Model file for the job. Use its own axes, mm. A direction names the side the tool comes from. Round coordinates to 2 decimals unless told otherwise and drop trailing zeros. Write each loop counter-clockwise with the first axis right and the second up, starting at its lowest first coordinate (ties: lowest second). Pieces come first, ordered by that corner, then holes. Notation, with made-up numbers: (52.5, 71.25) - (57.5, 71.25) arc R13 ccw to (57.5, 94.25) - close; hole circle Ø11 at (12, 2.25). An arc over 180 degrees is marked (long way). One line per item, written item: value.
from build123d import *

# Parameters (mm, degrees)
SKETCH1_R           = 3.4925
BOSS_EXTRUDE1_DEPTH = 25.4
SKETCH2_R           = 1.778
CUT_EXTRUDE1_DEPTH  = 54.415541746
FILLET2_R           = 6.35
FILLET1_R           = 6.35


with BuildPart() as part:
    # Sketch1 → Boss-Extrude1 (new body)
    with BuildSketch(Plane.XY):
        Polygon((0, 0), (44.45, 0), (44.45, 6.35), (31.75, 6.35), (31.75, 21.59), (12.7, 21.59), (12.7, 6.35), (0, 6.35), align=None)
        with Locations((22.225, 13.97)):
            Circle(SKETCH1_R, mode=Mode.SUBTRACT)
    extrude(amount=BOSS_EXTRUDE1_DEPTH)

    # Sketch2 → Cut-Extrude1 (cut, through all)
    with BuildSketch(Plane(origin=(0, 6.35, 0), x_dir=(1, 0, 0), z_dir=(0, 1, 0))):
        with Locations(Location((6.35, -6.35, 0), (0, 0, 270))):
            Circle(SKETCH2_R)
        with Locations(Location((6.35, -19.05, 0), (0, 0, 270))):
            Circle(SKETCH2_R)
        with Locations(Location((38.1, -6.35, 0), (0, 0, 270))):
            Circle(SKETCH2_R)
        with Locations(Location((38.1, -19.05, 0), (0, 0, 270))):
            Circle(SKETCH2_R)
    extrude(amount=-CUT_EXTRUDE1_DEPTH, mode=Mode.SUBTRACT)

    # Fillet2
    fillet2_edges = [part.edges().sort_by_distance(p)[0] for p in [
        (12.7, 21.59, 12.7),
        (31.75, 21.59, 12.7),
    ]]
    fillet(fillet2_edges, radius=FILLET2_R)

    # Fillet1
    fillet1_edges = [part.edges().sort_by_distance(p)[0] for p in [
        (44.45, 3.175, 0),
        (0, 3.175, 0),
        (44.45, 3.175, 25.4),
        (0, 3.175, 25.4),
    ]]
    fillet(fillet1_edges, radius=FILLET1_R)


solid = part.part
1. Wall check: probe 1 along Z at (x, y) = (38, 1); probe 2 along X at (y, z) = (3.75, 6.35); probe 3 along Z at (x, y) = (5, 3.25). Give the ranges that are in metal, low to high. Write a range as [from, to].
Report:
probe 1: [0, 4.57], [8.13, 17.27], [20.83, 25.4]
probe 2: [0, 4.57], [8.13, 36.32], [39.88, 44.45]
probe 3: [0.15, 5.19], [7.51, 17.89], [20.21, 25.25]
2. Band-saw the part on D-D on x = 5.5. Write the cut outline in (y, z).
Report:
outline: (0, 0.06) - (6.35, 0.06) - (6.35, 4.79) - (0, 4.79) - close; (0, 7.91) - (6.35, 7.91) - (6.35, 17.49) - (0, 17.49) - close; (0, 20.61) - (6.35, 20.61) - (6.35, 25.34) - (0, 25.34) - close
3. Band-saw the part on A-A on y = 13.97. Write the cut outline in (x, z), plus the area to 3 significant figures.
Report:
outline: (12.7, 0) - (18.73, 0) - (18.73, 25.4) - (12.7, 25.4) - close; (25.72, 0) - (31.75, 0) - (31.75, 25.4) - (25.72, 25.4) - close
area: 306 mm²
4. Tool access for faces 4 (the face through (22, 0, 13)), 5 (the face through (31.75, 11, 13)), 6 (the face through (6, 6.35, 13)): list every direction of +Z, -Z, +X, -X, +Y, -Y with a clear straight run to the whole face (end or side of a thin tool).
Report:
face 4: +Z, -Z, +X, -X, -Y
face 5: +Z, -Z, +X, +Y
face 6: +Z, -Z, -X, +Y
5. Band-saw the part on C-C on y = 4. Write the cut outline in (x, z).
Report:
outline: (0, 6.35) arc R6.35 ccw to (6.35, 0) - (38.1, 0) arc R6.35 ccw to (44.45, 6.35) - (44.45, 19.05) arc R6.35 ccw to (38.1, 25.4) - (6.35, 25.4) arc R6.35 ccw to (0, 19.05) - close; hole circle Ø3.56 at (6.35, 6.35); hole circle Ø3.56 at (6.35, 19.05); hole circle Ø3.56 at (38.1, 6.35); hole circle Ø3.56 at (38.1, 19.05)
6. Mould opens along Y. For faces 1 (the face through (42.54, 3.22, 1.81)), 2 (the face through (18.736, 14.124, 12.522)), 3 (the face through (38, 6.35, 13)) say: released by +Y, released by -Y, zero draft, split by the parting line, or undercut.
Report:
face 1: zero draft
face 2: undercut
face 3: released by +Y
7. Drop flat-ended pins along their axis: pin 1 (1.5 mm diameter, centred on y = 17.5, z = 13.5, fed in from +X); pin 2 (10 mm diameter, centred on x = 7.5, z = 15, fed in from +Y); pin 3 (8 mm diameter, centred on y = 10, z = 3, fed in from +X). Give the stop position or say it passes through.
Report:
pin 1: x = 31.57
pin 2: y = 6.35
pin 3: x = 44.21
